Geometry check sheet. Reference: the model listing, model coordinates, mm. A direction names the side the tool comes from. Coordinates: 2 decimals unless noted, no trailing zeros. Order: outer loops, then holes, each group sorted by start corner. A loop starts at its lowest first (then second) coordinate and runs counter-clockwise, first axis right, second up. Notation, with made-up numbers: (-32, 78) -> (9, 78) arc R18 ccw to (9, 110) -> close; hole circle Ø11 at (68, 38). An arc over 180 degrees is marked (long way). Answer as CSV lines item,"result". Start each with the question number.
from build123d import *

# Parameters (mm, degrees)
F0_W        = 88.9
F0_H        = 165.1
F1_DEPTH    = 6.35
F2_DEPTH    = 50.8
F3_DEPTH    = 25.4
F4_R        = 6.34999
F5_C1_SIZE2 = 12.7
F5_C1_SIZE  = 7.3323484187
F5_C2_SIZE2 = 12.7
F5_C2_SIZE  = 7.3323484187
F5_C3_SIZE2 = 7.3323484187
F5_C3_SIZE  = 12.7
F5_C4_SIZE2 = 12.7
F5_C4_SIZE  = 7.3323484187
F5_C5_SIZE2 = 7.3323484187
F5_C5_SIZE  = 12.7
F5_C6_SIZE2 = 7.3323484187
F5_C6_SIZE  = 12.7
F6_SIZE2    = 7.3323484187
F6_SIZE     = 12.7


# Not quite as in the source:
# - a fillet or chamfer is up to 0.001 mm smaller than in the source, because OpenCascade refuses the exact size


with BuildPart() as f1:
    # F0 (on Top) → F1 (new body)
    with BuildSketch(Plane.XY):
        with Locations((0, -32.9789540072)):
            Rectangle(F0_W, F0_H)
        Polygon((-38.1, 5.1210459928), (-38.1, 43.2210459928), (0, 43.2210459928), (38.1, 43.2210459928), (38.1, -71.0789540072), (38.1, -109.1789540072), (0, -109.1789540072), (-38.1, -109.1789540072), align=None, mode=Mode.SUBTRACT)
    extrude(amount=F1_DEPTH)

    # F0 (on Top) → F2 (join)
    with BuildSketch(Plane.XY):
        with BuildLine():
            Line((0, 43.2210459928), (-38.1, 43.2210459928))
            Line((-38.1, 43.2210459928), (-38.1, 5.1210459928))
            Line((-38.1, 5.1210459928), (-12.7, 5.1210459928))
            ThreePointArc((-12.7, 5.1210459928), (-3.7197438789, 8.8407898717), (0, 17.8210459928))
            Line((0, 17.8210459928), (0, 43.2210459928))
        make_face()
        with BuildLine():
            Line((38.1, -109.1789540072), (38.1, -71.0789540072))
            Line((38.1, -71.0789540072), (12.7, -71.0789540072))
            ThreePointArc((12.7, -71.0789540072), (3.7197438789, -74.7986978861), (0, -83.7789540072))
            Line((0, -83.7789540072), (0, -109.1789540072))
            Line((0, -109.1789540072), (38.1, -109.1789540072))
        make_face()
    extrude(amount=F2_DEPTH)

    # F0 (on Top) → F3 (join)
    with BuildSketch(Plane.XY):
        with BuildLine():
            Line((38.1, 43.2210459928), (0, 43.2210459928))
            Line((0, 43.2210459928), (0, 17.8210459928))
            ThreePointArc((0, 17.8210459928), (-3.7197438789, 8.8407898717), (-12.7, 5.1210459928))
            Line((-12.7, 5.1210459928), (-38.1, 5.1210459928))
            Line((-38.1, 5.1210459928), (-38.1, -109.1789540072))
            Line((-38.1, -109.1789540072), (0, -109.1789540072))
            Line((0, -109.1789540072), (0, -83.7789540072))
            ThreePointArc((0, -83.7789540072), (3.7197438789, -74.7986978861), (12.7, -71.0789540072))
            Line((12.7, -71.0789540072), (38.1, -71.0789540072))
            Line((38.1, -71.0789540072), (38.1, 43.2210459928))
        make_face()
    extrude(amount=F3_DEPTH)

    # F4 (radius 6.35 in the source; OpenCascade refuses exactly that, so slightly less here)
    f4_edges = [f1.edges().sort_by_distance(p)[0] for p in [
        (44.45, -32.978954, 6.35),
        (0, 49.571046, 6.35),
        (0, -115.528954, 6.35),
        (-44.45, -32.978954, 6.35),
    ]]
    fillet(f4_edges, radius=F4_R)

    # F5: chamfer of 12.7 x 7.3323484187 on 6 edges, made by hand

    # F5_c1
    f5_c1_edges = [f1.edges().sort_by_distance(p)[0] for p in [
        (-38.1, 24.1710459928, 50.8),
    ]]
    f5_c1_side = f1.faces().sort_by_distance((-38.1, 24.1710459928, 50.6533530316))[0]
    chamfer(f5_c1_edges, length=F5_C1_SIZE, length2=F5_C1_SIZE2, reference=f5_c1_side)

    # F5_c2
    f5_c2_edges = [f1.edges().sort_by_distance(p)[0] for p in [
        (-38.1, -52.0289540072, 25.4),
    ]]
    f5_c2_side = f1.faces().sort_by_distance((-38.1, -52.0289540072, 25.2533530316))[0]
    chamfer(f5_c2_edges, length=F5_C2_SIZE, length2=F5_C2_SIZE2, reference=f5_c2_side)

    # F5_c3
    f5_c3_edges = [f1.edges().sort_by_distance(p)[0] for p in [
        (19.05, 43.2210459928, 25.4),
    ]]
    f5_c3_side = f1.faces().sort_by_distance((19.05, 43.2210459928, 25.2533530316))[0]
    chamfer(f5_c3_edges, length=F5_C3_SIZE, length2=F5_C3_SIZE2, reference=f5_c3_side)

    # F5_c4
    f5_c4_edges = [f1.edges().sort_by_distance(p)[0] for p in [
        (-12.7, 43.2210459928, 50.8),
    ]]
    f5_c4_side = f1.faces().sort_by_distance((-12.7, 43.2210459928, 50.6533530316))[0]
    chamfer(f5_c4_edges, length=F5_C4_SIZE, length2=F5_C4_SIZE2, reference=f5_c4_side)

    # F5_c5
    f5_c5_edges = [f1.edges().sort_by_distance(p)[0] for p in [
        (38.1, -17.5951282165, 25.4),
    ]]
    f5_c5_side = f1.faces().sort_by_distance((38.1, -17.5951282165, 25.2533530316))[0]
    chamfer(f5_c5_edges, length=F5_C5_SIZE, length2=F5_C5_SIZE2, reference=f5_c5_side)

    # F5_c6
    f5_c6_edges = [f1.edges().sort_by_distance(p)[0] for p in [
        (-12.7, -109.1789540072, 25.4),
    ]]
    f5_c6_side = f1.faces().sort_by_distance((-12.7, -109.0323070388, 25.4))[0]
    chamfer(f5_c6_edges, length=F5_C6_SIZE, length2=F5_C6_SIZE2, reference=f5_c6_side)

    # F6
    f6_edges = [f1.edges().sort_by_distance(p)[0] for p in [
        (19.05, -109.178954, 50.8),
        (38.1, -90.128954, 50.8),
    ]]
    f6_side = f1.faces().sort_by_distance((19.446042, -90.524996, 50.8))[0]
    chamfer(f6_edges, length=F6_SIZE, length2=F6_SIZE2, reference=f6_side)


solid = f1.part
Q1. Go/stop test with flat-tipped pins: pin 1 Ø12.5 at (x, z) = (23, 26.5) entering from +Y; pin 2 Ø10 at (x, y) = (-1, -57) entering from +Z; pin 3 Ø2 at (y, z) = (4.5, 40) entering from -X; pin 4 Ø1 at (x, y) = (-8, -15.5) entering from -Z. Record where each tip stops, or that it passes through.
Q2. Release check for a two-part mould opening along Z. For faces 6 (the flat face through (0, -96, 38)), 7 (the cylindrical face through (0.62, -113.62, 4.54)) record: released by +Z, released by -Z, zero draft, split by the parting line, or undercut.
Q3. Sectioned sample at A-A, the plane z = 32.5. Record the cut outline in (x, y), then the cut area to 3 significant figures.
Q4. Access from +Z, -Z, +X, -X, +Y, -Y to the whole of each face (thin tool, end or side, straight path). Record for faces 1 (the flat face through (38.1, -68, 12)), 2 (the flat face through (0, 30, 36)), 3 (the flat face through (8, -109.179, 21)), 4 (the flat face through (-31.661, 20.204, 47.185)), 5 (the flat face through (-14.55, 36.782, 47.185)).
Q5. Thickness scan on L1, parallel to Z at x = 11.5, y = -12; L2, parallel to X at y = -103, z = 13; L3, parallel to X at y = -96, z = 40. Record the ranges inside material, lowest first.
Geometry results:
1,pin 1,"stops at y = 38.86"
1,pin 2,"stops at z = 25.4"
1,pin 3,"stops at x = -38.1"
1,pin 4,"stops at z = 0"
2,face 6,"zero draft"
2,face 7,"released by +Z"
3,outline,"(-38.1, 5.12) -> (-12.7, 5.12) arc R12.7 ccw to (0, 17.82) -> (0, 43.22) -> (-38.1, 43.22) -> close; (0, -109.18) -> (38.1, -109.18) -> (38.1, -71.08) -> (12.7, -71.08) arc R12.7 ccw to (0, -83.78) -> close"
3,area,"2,830 mm^2"
4,face 1,"+Z, +X, +Y, -Y"
4,face 2,"+Z, +X, +Y"
4,face 3,"+Z, +X, -X, -Y"
4,face 4,"+Z, -X, +Y, -Y"
4,face 5,"+Z, +X, -X, +Y"
5,L1,"z = 0 to 25.4"
5,L2,"x = -38.1 to 38.1"
5,L3,"x = 0 to 38.1"
